Could you check a few things on this drawing? It's one solid part, dimensions in mm from its lowest x, y, z. A direction names the side the tool comes from. Give positions to 0.01 mm unless a question says otherwise; leave off trailing zeros. Order: outer loops, then holes, each group sorted by start corner. A loop starts at its lowest first (then second) coordinate and runs counter-clockwise, first axis right, second up.
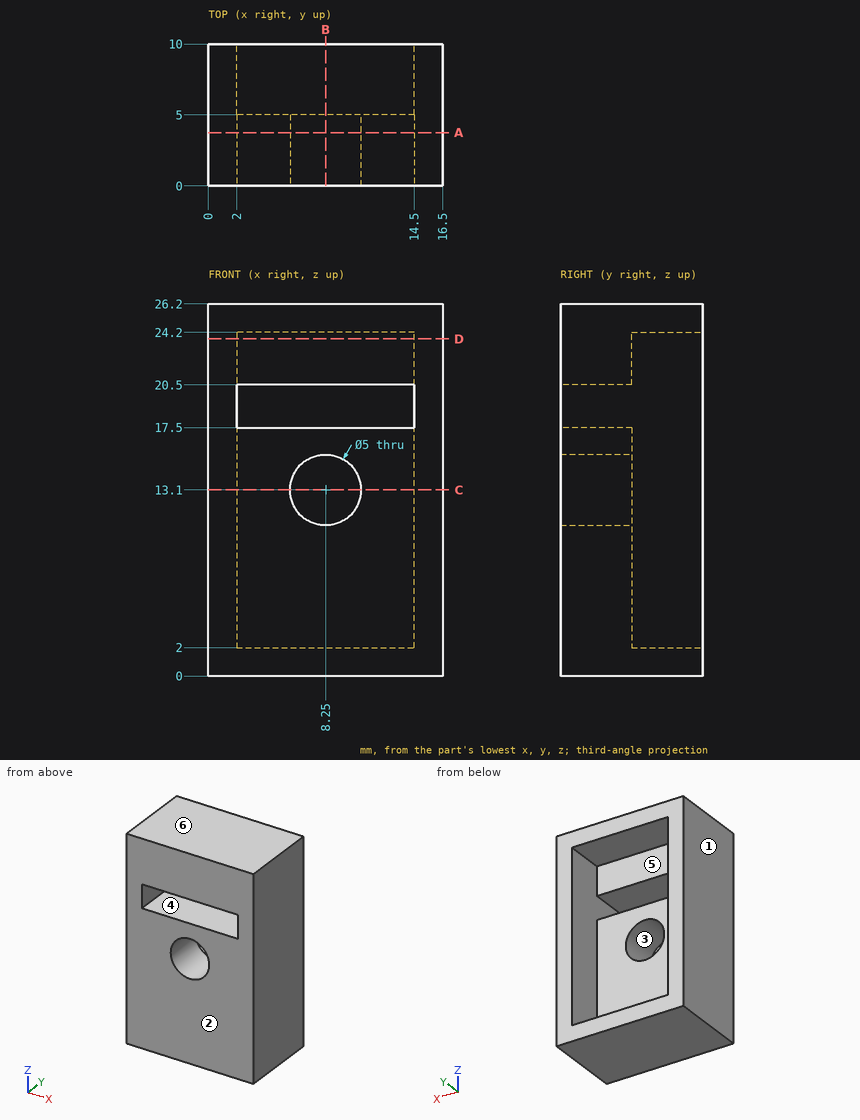
Item 1: For the marked faces 4, 5 and 6, which set-ups out of +Z, -Z, +X, -X, +Y, -Y let a thin tool reach every point of the face, with its end or its side?
Findings:
face 4: +Y, -Y
face 5: +Y
face 6: +Z, +X, -X, +Y, -Y
Item 2: Imagine slicing it at D-D on z = 23.75. List the corners of the cut face in (x, y) for me.
Findings:
outline: (0, 0) - (16.5, 0) - (16.5, 10) - (14.5, 10) - (14.5, 5) - (2, 5) - (2, 10) - (0, 10) - close
Item 3: Please list where these lines run through material, in increasing order: line 1 along Z through (x, y) = (8.25, 2.55); line 2 along Z through (x, y) = (2.5, 5.25); line 3 along X through (y, z) = (4.25, 19.25).
Findings:
line 1: z = 0 to 10.6, 15.6 to 17.5, 20.5 to 26.2
line 2: z = 0 to 2, 24.2 to 26.2
line 3: x = 0 to 2, 14.5 to 16.5
Item 4: Imagine slicing it at C-C on z = 13.1. List the corners of the cut face in (x, y) for me, then the cut area to 3 significant figures.
Findings:
outline: (0, 0) - (5.75, 0) - (5.75, 5) - (2, 5) - (2, 10) - (0, 10) - close; (10.75, 0) - (16.5, 0) - (16.5, 10) - (14.5, 10) - (14.5, 5) - (10.75, 5) - close
area: 77.5 mm2
Item 5: For pin 1 (1.8 mm diameter, centred on x = 7.5, z = 22.5, fed in from +Y), with a flat end and sliding along its axis, tell me the tip position at first contact or that it passes through.
Findings:
pin 1: stops at y = 5
Item 6: Imagine slicing it at A-A on y = 3.75. List the corners of the cut face in (x, z) for me, then the cut area to 3 significant figures.
Findings:
outline: (0, 0) - (16.5, 0) - (16.5, 26.2) - (0, 26.2) - close; hole (2, 17.5) - (14.5, 17.5) - (14.5, 20.5) - (2, 20.5) - close; hole circle Ø5 at (8.25, 13.1)
area: 375 mm2
Item 7: We'd pull the mould along X, two halves only. Please class the marked faces 1, 2 and 3: +X half, -X half, draft (parallel to the pull), parting line (faces both ways), or undercut.
Findings:
face 1: -X half
face 2: draft
face 3: undercut
Item 8: Imagine slicing it at B-B on x = 8.25. List the corners of the cut face in (y, z) for me.
Findings:
outline: (0, 0) - (10, 0) - (10, 2) - (5, 2) - (5, 10.6) - (0, 10.6) - close; (0, 15.6) - (5, 15.6) - (5, 17.5) - (0, 17.5) - close; (0, 20.5) - (5, 20.5) - (5, 24.2) - (10, 24.2) - (10, 26.2) - (0, 26.2) - close
